Design review of the part built by this model. Coordinates are the model's own, in mm. A direction names the side the tool comes from. Give positions to 0.01 mm unless a question says otherwise; leave off trailing zeros. Write each loop counter-clockwise with the first axis right and the second up, starting at its lowest first coordinate (ties: lowest second). Pieces come first, ordered by that corner, then holes. Notation, with made-up numbers: M 76.5,-13 L 105.5,-13 A10 ccw 105.5,5 Z; hole C 19,25.5 d4. An arc over 180 degrees is marked long. Answer in a Markdown table with one row per item.
Autodesk Fusion 360 part; units mm, degrees
sketch "Sketch1" plane through (0, 0, 0) normal (0, 0, 1) x (1, 0, 0)
  line L0 (4, 0) -> (56.35, 0)
  line L1 (60.35, 4) -> (60.35, 83.39)
  line L2 (56.35, 87.39) -> (4, 87.39)
  line L3 (0, 83.39) -> (0, 4)
  arc A0 (4, 87.39) -> (0, 83.39) centre (4, 83.39) ccw
  arc A1 (60.35, 83.39) -> (56.35, 87.39) centre (56.35, 83.39) ccw
  arc A2 (56.35, 0) -> (60.35, 4) centre (56.35, 4) ccw
  arc A3 (0, 4) -> (4, 0) centre (4, 4) ccw
  line L4 (30.175, 81.69) -> (25.475, 81.69)
  line L5 (30.175, 81.69) -> (34.875, 81.69)
  line L6 (30.175, 77.39) -> (25.475, 77.39)
  line L7 (30.175, 77.39) -> (34.875, 77.39)
  line L8 (25.475, 81.69) -> (25.475, 77.39)
  line L9 (34.875, 81.69) -> (34.875, 77.39)
  line L10 (34.875, 66.4941) -> (25.475, 66.4941)
  line L11 (34.875, 57.0941) -> (25.475, 57.0941)
  line L12 (34.875, 57.0941) -> (34.875, 61.7941)
  line L13 (34.875, 61.7941) -> (34.875, 66.4941)
  line L14 (25.475, 57.0941) -> (25.475, 61.7941)
  line L15 (25.475, 61.7941) -> (25.475, 66.4941)
  point P0 (60.35, 0)
  point P1 (0, 87.39)
  dimension "d6" = 60.35
  dimension "d7" = 87.39
  dimension "d9" = 4
  dimension "d10" = 4
  dimension "d11" = 4
  dimension "d12" = 4
  dimension "d16" = 4.3
extrude "Extrude2" add sketch "Sketch1" along normal blind 4.6
extrude "Extrude1" [suppressed]
equation "long_side_length = 87.39 mm"
equation "short_side_length = 60.35 mm"
equation "kerf = 0.6 mm"
equation "notch_depth = 10 mm"
equation "thickness = 4.6 mm"
equation "d6 = short_side_length"
equation "d7 = long_side_length"
equation "rounded_edge_length = 4 mm"
equation "d9 = rounded_edge_length"
equation "d10 = rounded_edge_length"
equation "d11 = rounded_edge_length"
equation "d12 = rounded_edge_length"
equation "d16 = thickness - ( kerf / 2 )"
equation "d22 = thickness"
equation "d43 = thickness"
1) The part is to be moulded in two halves that separate along X. For faces 1 (the face through (1.203, 1.141, 2.268)), 2 (the face through (30, 44, 0)), 3 (the face through (30, 57.094, 2)), 4 (the face through (30, 66.494, 2)), say which applies: released by +X, released by -X, zero draft, split by the parting line, or undercut.
Geometry says:
| item | result |
|---|---|
| face 1 | released by -X |
| face 2 | zero draft |
| face 3 | undercut |
| face 4 | undercut |
2) Add section A-A (z = 1.8). Write out the cut boundary in (x, y) (3 decimals), and give its area (3 significant figures).
Geometry says:
| item | result |
|---|---|
| outline | M 0,4 A4 ccw 4,0 L 56.35,0 A4 ccw 60.35,4 L 60.35,83.39 A4 ccw 56.35,87.39 L 4,87.39 A4 ccw 0,83.39 Z; hole M 25.475,57.094 L 34.875,57.094 L 34.875,66.494 L 25.475,66.494 Z; hole M 25.475,77.39 L 34.875,77.39 L 34.875,81.69 L 25.475,81.69 Z |
| area | 5,130 mm^2 |
3) Add section B-B (x = 31.5). Write out the cut boundary in (y, z), and give its area (3 significant figures).
Geometry says:
| item | result |
|---|---|
| outline | M 0,0 L 57.09,0 L 57.09,4.6 L 0,4.6 Z; M 66.49,0 L 77.39,0 L 77.39,4.6 L 66.49,4.6 Z; M 81.69,0 L 87.39,0 L 87.39,4.6 L 81.69,4.6 Z |
| area | 339 mm^2 |
4) To check wall thickness, follow probe 1 along Y at (x, z) = (29, 3.8); probe 2 along X at (y, z) = (81.5, 0.55) (3 decimals). State the ranges of each line that lie inside material, in increasing order. Write a range as [from, to].
Geometry says:
| item | result |
|---|---|
| probe 1 | [0, 57.09], [66.49, 77.39], [81.69, 87.39] |
| probe 2 | [0, 25.475], [34.875, 60.35] |
5) For faces 5 (the face through (30, 81.69, 2)), 6 (the face through (1.141, 86.187, 2.268)), list the 3-axis set-ups (+Z, -Z, +X, -X, +Y, -Y) from which the entire face can be reached by the end or side of a thin tool; tool diameter is ignored.
Geometry says:
| item | result |
|---|---|
| face 5 | +Z, -Z |
| face 6 | +Z, -Z, -X, +Y |
